Geometry check sheet. Reference: the model listing, model coordinates, mm. Round coordinates to 2 decimals unless told otherwise and drop trailing zeros. Write each loop counter-clockwise with the first axis right and the second up, starting at its lowest first coordinate (ties: lowest second). Pieces come first, ordered by that corner, then holes. Notation, with made-up numbers: M 68.5,87 L 110.5,87 A27 ccw 110.5,112 Z; hole C -1,42.25 d6. An arc over 180 degrees is marked long. One line per item, written item: value. Start each with the question number.
1. Section check D-D (x = 7.5). Record the boundary of the cut face in (y, z).
2. Scan lines: probe 1 along Z at (x, y) = (-7, -1.75); probe 2 along X at (y, z) = (-0.45, -2.5); probe 3 along X at (y, z) = (-0.8, 0.5). Record each from-to range of solid material in increasing order. Write a range as [from, to].
3. Depth check by flat-ended pin: P1, Ø0.6, axis at x = -17.5, y = -4.5, coming from the +Z side; P2, Ø1.5, axis at y = -3.5, z = -8.5, coming from the +X side; P3, Ø1.6, axis at x = 0, z = 1, coming from the +Y side (3 decimals); P4, Ø1, axis at y = -3.5, z = 17.5, coming from the +X side. Enter the tip coordinate at first touch or a pass-through.
4. Section check A-A (z = 0). Count the separate pieces of the cut face and the enclosed holes in it, and give its area (3 significant figures).
from build123d import *

# Parameters (mm, degrees)
F0_R     = 16.75
F1_DEPTH = 5
F3_DEPTH = 2
F4_R     = 2
F5_DEPTH = 5
F6_R     = 2.8491120017
F6_R_2   = 3
F6_R_3   = 2.9757166717
F6_R_4   = 2.5074273039
F6_R_5   = 2.7276966812
F6_R_6   = 2.9574204399
F7_DEPTH = 1.5
F8_R     = 0.5


with BuildPart() as f1:
    # F0 (on Front) → F1 (new body)
    with BuildSketch(Plane.XZ):
        Circle(F0_R)
    extrude(amount=F1_DEPTH)

    # F2 (on face) → F3 (join)
    with BuildSketch(Plane.XZ.offset(5)):
        with BuildLine():
            Line((5.2447166905, 15.9077165815), (5.2447166905, 19.3000763428))
            ThreePointArc((5.2447166905, 19.3000763428), (-0.5802396301, 19.9915812774), (-6.3552833095, 18.9633956362))
            Line((-6.3552833095, 18.9633956362), (-6.3552833095, 15.4975118666))
            ThreePointArc((-6.3552833095, 15.4975118666), (-0.5919514598, 16.7395368356), (5.2447166905, 15.9077165815))
        make_face()
        with BuildLine():
            ThreePointArc((15.4975118666, 6.3552833095), (11.418067119, 12.2552129017), (5.2447166905, 15.9077165815))
            ThreePointArc((5.2447166905, 15.9077165815), (-0.5919514598, 16.7395368356), (-6.3552833095, 15.4975118666))
            ThreePointArc((-6.3552833095, 15.4975118666), (-12.2552129017, 11.418067119), (-15.9077165815, 5.2447166905))
            ThreePointArc((-15.9077165815, 5.2447166905), (-16.7395368356, -0.5919514598), (-15.4975118666, -6.3552833095))
            ThreePointArc((-15.4975118666, -6.3552833095), (-11.418067119, -12.2552129017), (-5.2447166905, -15.9077165815))
            ThreePointArc((-5.2447166905, -15.9077165815), (0.5919514598, -16.7395368356), (6.3552833095, -15.4975118666))
            ThreePointArc((6.3552833095, -15.4975118666), (12.2552129017, -11.418067119), (15.9077165815, -5.2447166905))
            ThreePointArc((15.9077165815, -5.2447166905), (16.5380886553, -2.6559600205), (16.75, 0))
            ThreePointArc((16.75, 0), (16.4338952133, 3.2387633623), (15.4975118666, 6.3552833095))
        make_face()
        with BuildLine():
            Line((18.9633956362, 6.3552833095), (15.4975118666, 6.3552833095))
            ThreePointArc((15.4975118666, 6.3552833095), (16.4338952133, 3.2387633623), (16.75, 0))
            ThreePointArc((16.75, 0), (16.5380886553, -2.6559600205), (15.9077165815, -5.2447166905))
            Line((15.9077165815, -5.2447166905), (19.3000763428, -5.2447166905))
            ThreePointArc((19.3000763428, -5.2447166905), (19.9915812774, 0.5802396301), (18.9633956362, 6.3552833095))
        make_face()
        with BuildLine():
            ThreePointArc((-15.4975118666, -6.3552833095), (-16.7395368356, -0.5919514598), (-15.9077165815, 5.2447166905))
            Line((-15.9077165815, 5.2447166905), (-19.3000763428, 5.2447166905))
            ThreePointArc((-19.3000763428, 5.2447166905), (-19.9915812774, -0.5802396301), (-18.9633956362, -6.3552833095))
            Line((-18.9633956362, -6.3552833095), (-15.4975118666, -6.3552833095))
        make_face()
        with BuildLine():
            ThreePointArc((6.3552833095, -15.4975118666), (0.5919514598, -16.7395368356), (-5.2447166905, -15.9077165815))
            Line((-5.2447166905, -15.9077165815), (-5.2447166905, -19.3000763428))
            ThreePointArc((-5.2447166905, -19.3000763428), (0.5802396301, -19.9915812774), (6.3552833095, -18.9633956362))
            Line((6.3552833095, -18.9633956362), (6.3552833095, -15.4975118666))
        make_face()
    extrude(amount=-F3_DEPTH)

    # F4 (on face) → F5 (cut, through all)
    with BuildSketch(Plane(origin=(0, 0, 0), x_dir=(-1, 0, 0), z_dir=(0, 1, 0))):
        with Locations((-7.7781745931, 7.7781745931)):
            Circle(F4_R)
        with Locations((-11, 0)):
            Circle(F4_R)
        with Locations((-7.7781745931, -7.7781745931)):
            Circle(F4_R)
        with Locations((0, -11)):
            Circle(F4_R)
        with Locations((7.7781745931, -7.7781745931)):
            Circle(F4_R)
        with Locations((11, 0)):
            Circle(F4_R)
        with Locations((7.7781745931, 7.7781745931)):
            Circle(F4_R)
        Circle(F4_R)
        with Locations((0, 11)):
            Circle(F4_R)
    extrude(amount=-F5_DEPTH, mode=Mode.SUBTRACT)

    # F6 (on face) → F7 (cut)
    with BuildSketch(Plane(origin=(0, 0, 0), x_dir=(-1, 0, 0), z_dir=(0, 1, 0))):
        with Locations((-7.7781745931, 7.7781745931)):
            Circle(F6_R)
        with Locations((-11, 0)):
            Circle(F6_R_2)
        with Locations((-7.7781745931, -7.7781745931)):
            Circle(F6_R_2)
        with Locations((0, -11)):
            Circle(F6_R_3)
        with Locations((7.7781745931, -7.7781745931)):
            Circle(F6_R_4)
        with Locations((11, 0)):
            Circle(F6_R_2)
        Circle(F6_R_5)
        with Locations((7.7781745931, 7.7781745931)):
            Circle(F6_R_6)
        with Locations((0, 11)):
            Circle(F6_R_2)
    extrude(amount=-F7_DEPTH, mode=Mode.SUBTRACT)

    # F8
    f8_edges = [f1.edges().sort_by_distance(p)[0] for p in [
        (5.244717, -4, 19.300076),
        (-6.355283, -4, 18.963396),
        (18.963396, -4, 6.355283),
        (-19.300076, -4, 5.244717),
        (19.300076, -4, -5.244717),
        (-18.963396, -4, -6.355283),
        (6.355283, -4, -18.963396),
        (-5.244717, -4, -19.300076),
    ]]
    fillet(f8_edges, radius=F8_R)


solid = f1.part
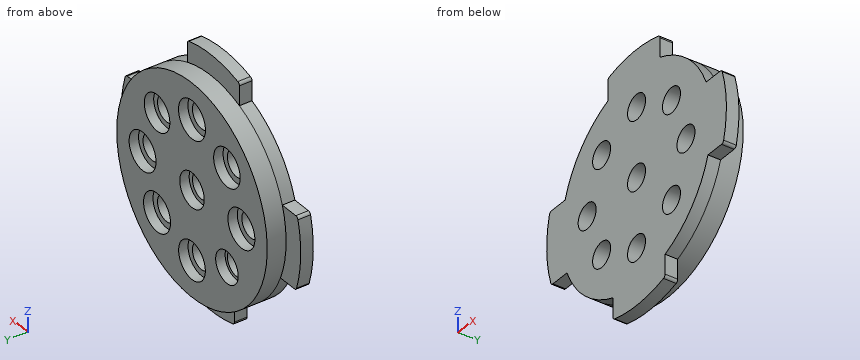
Result sheet:
1. outline: M -5,-14.98 L 0,-14.98 L 0,-10.77 L -1.5,-10.77 L -1.5,-9.76 L -5,-9.76 Z; M -5,-5.8 L -1.5,-5.8 L -1.5,-4.79 L 0,-4.79 L 0,4.94 L -1.5,4.94 L -1.5,5.8 L -5,5.8 Z; M -5,9.76 L -1.5,9.76 L -1.5,10.61 L 0,10.61 L 0,14.98 L -5,14.98 Z
2. probe 1: z = [-15.22, -9.62], [-5.94, 5.94], [9.62, 15.22]
2. probe 2: x = [-16.56, -12.66], [-9.34, -1.09], [1.09, 9.34], [12.66, 16.56]
2. probe 3: x = [-16.74, -13.96], [-8.04, -2.68], [2.68, 8.04], [13.96, 16.74]
3. P1: stops at z = 5.24
3. P2: stops at x = 14.85
3. P3: passes through
3. P4: stops at x = 5.24
4. separate pieces: 4
4. enclosed holes: 0
4. area: 112 mm2
